Geometry: final body of the model. Coordinates: model frame, mm. Round coordinates to 2 decimals unless told otherwise and drop trailing zeros. Loops run counter-clockwise (first coordinate to the right, second up) from the corner with the lowest first, then second, coordinate; pieces in that order, holes last. Notation, with made-up numbers: M 65,35 L 92,35 A18 cw 92,51 Z; hole C -34,35.25 d7. An arc over 180 degrees is marked long. Return JSON: item names as keys, results as strings.
from build123d import *

# Parameters (mm, degrees)
F1_DEPTH  = 4
F3_DEPTH  = 2
F5_DEPTH  = 2
F6_W      = 5
F6_H      = 4
F6_W_2    = 4
F6_H_2    = 5
F7_DEPTH  = 2
F9_R      = 5
F10_DEPTH = 4.001


with BuildPart() as f1:
    # F0 (on Top) → F1 (new body)
    with BuildSketch(Plane.XY):
        with BuildLine():
            ThreePointArc((51.5, 24), (48.5710678119, 31.0710678119), (41.5, 34))
            Line((41.5, 34), (-41.5, 34))
            ThreePointArc((-41.5, 34), (-48.5710678119, 31.0710678119), (-51.5, 24))
            Line((-51.5, 24), (-51.5, -24))
            ThreePointArc((-51.5, -24), (-48.5710678119, -31.0710678119), (-41.5, -34))
            Line((-41.5, -34), (41.5, -34))
            ThreePointArc((41.5, -34), (48.5710678119, -31.0710678119), (51.5, -24))
            Line((51.5, -24), (51.5, 24))
        make_face()
        with BuildLine():
            ThreePointArc((41.5, 30), (45.7426406871, 28.2426406871), (47.5, 24))
            Line((47.5, 24), (47.5, -24))
            ThreePointArc((47.5, -24), (45.7426406871, -28.2426406871), (41.5, -30))
            Line((41.5, -30), (-41.5, -30))
            ThreePointArc((-41.5, -30), (-45.7426406871, -28.2426406871), (-47.5, -24))
            Line((-47.5, -24), (-47.5, 24))
            ThreePointArc((-47.5, 24), (-45.7426406871, 28.2426406871), (-41.5, 30))
            Line((-41.5, 30), (41.5, 30))
        make_face(mode=Mode.SUBTRACT)
    extrude(amount=F1_DEPTH)

    # F2 (on face) → F5 (join)
    with BuildSketch(Plane.XY.offset(4)):
        with BuildLine():
            ThreePointArc((51.5, 24), (48.5710678119, 31.0710678119), (41.5, 34))
            Line((41.5, 34), (-41.5, 34))
            ThreePointArc((-41.5, 34), (-48.5710678119, 31.0710678119), (-51.5, 24))
            Line((-51.5, 24), (-51.5, -24))
            ThreePointArc((-51.5, -24), (-48.5710678119, -31.0710678119), (-41.5, -34))
            Line((-41.5, -34), (41.5, -34))
            ThreePointArc((41.5, -34), (48.5710678119, -31.0710678119), (51.5, -24))
            Line((51.5, -24), (51.5, 24))
        make_face()
        with BuildLine():
            Line((-41.5, 30), (41.5, 30))
            ThreePointArc((41.5, 30), (45.7426406871, 28.2426406871), (47.5, 24))
            Line((47.5, 24), (47.5, -24))
            ThreePointArc((47.5, -24), (45.7426406871, -28.2426406871), (41.5, -30))
            Line((41.5, -30), (-41.5, -30))
            ThreePointArc((-41.5, -30), (-45.7426406871, -28.2426406871), (-47.5, -24))
            Line((-47.5, -24), (-47.5, 24))
            ThreePointArc((-47.5, 24), (-45.7426406871, 28.2426406871), (-41.5, 30))
        make_face(mode=Mode.SUBTRACT)
        with BuildLine():
            ThreePointArc((47.5, 24), (45.7426406871, 28.2426406871), (41.5, 30))
            Line((41.5, 30), (-41.5, 30))
            ThreePointArc((-41.5, 30), (-45.7426406871, 28.2426406871), (-47.5, 24))
            Line((-47.5, 24), (-47.5, -24))
            ThreePointArc((-47.5, -24), (-45.7426406871, -28.2426406871), (-41.5, -30))
            Line((-41.5, -30), (41.5, -30))
            ThreePointArc((41.5, -30), (45.7426406871, -28.2426406871), (47.5, -24))
            Line((47.5, -24), (47.5, 24))
        make_face()
    extrude(amount=-F5_DEPTH)

    # F6 (on face) → F7 (cut)
    with BuildSketch(Plane(origin=(0, 0, 0), x_dir=(1, 0, 0), z_dir=(0, 0, -1))):
        with Locations((-35.85, 32)):
            Rectangle(F6_W, F6_H)
        with Locations((35.85, 32)):
            Rectangle(F6_W, F6_H)
        with Locations((-35.85, -32)):
            Rectangle(F6_W, F6_H)
        with Locations((35.85, -32)):
            Rectangle(F6_W, F6_H)
        with Locations((-49.5, 20)):
            Rectangle(F6_W_2, F6_H_2)
        with Locations((-49.5, -20)):
            Rectangle(F6_W_2, F6_H_2)
        with Locations((49.5, -20)):
            Rectangle(F6_W_2, F6_H_2)
        with Locations((49.5, 20)):
            Rectangle(F6_W_2, F6_H_2)
    extrude(amount=-F7_DEPTH, mode=Mode.SUBTRACT)

    # F9 (on face) → F10 (cut, through all)
    with BuildSketch(Plane.XY.offset(4)):
        with Locations((-42.4, 24)):
            Circle(F9_R)
        with BuildLine():
            Line((-26.8, 30), (-36.8, 30))
            ThreePointArc((-36.8, 30), (-31.8, 25), (-26.8, 30))
        make_face()
        with Locations((-31.8, 18)):
            Circle(F9_R)
        with Locations((-42.4, 12)):
            Circle(F9_R)
        with Locations((-42.4, 0)):
            Circle(F9_R)
        with Locations((-31.8, 6)):
            Circle(F9_R)
        with Locations((-31.8, -6)):
            Circle(F9_R)
        with Locations((-42.4, -12)):
            Circle(F9_R)
        with Locations((-42.4, -24)):
            Circle(F9_R)
        with Locations((-31.8, -18)):
            Circle(F9_R)
        with BuildLine():
            ThreePointArc((-26.8, -30), (-31.8, -25), (-36.8, -30))
            Line((-36.8, -30), (-26.8, -30))
        make_face()
        with Locations((-21.2, -24)):
            Circle(F9_R)
        with Locations((-21.2, -12)):
            Circle(F9_R)
        with Locations((-21.2, 0)):
            Circle(F9_R)
        with Locations((-21.2, 12)):
            Circle(F9_R)
        with Locations((-21.2, 24)):
            Circle(F9_R)
        with BuildLine():
            ThreePointArc((-15.6, 30), (-10.6, 25), (-5.6, 30))
            Line((-5.6, 30), (-15.6, 30))
        make_face()
        with Locations((-10.6, 18)):
            Circle(F9_R)
        with Locations((-10.6, 6)):
            Circle(F9_R)
        with Locations((-10.6, -6)):
            Circle(F9_R)
        with Locations((-10.6, -18)):
            Circle(F9_R)
        with BuildLine():
            Line((-15.6, -30), (-5.6, -30))
            ThreePointArc((-5.6, -30), (-10.6, -25), (-15.6, -30))
        make_face()
        with Locations((0, -24)):
            Circle(F9_R)
        with Locations((0, -12)):
            Circle(F9_R)
        Circle(F9_R)
        with Locations((0, 12)):
            Circle(F9_R)
        with Locations((0, 24)):
            Circle(F9_R)
        with BuildLine():
            Line((15.6, 30), (5.6, 30))
            ThreePointArc((5.6, 30), (10.6, 25), (15.6, 30))
        make_face()
        with Locations((10.6, 18)):
            Circle(F9_R)
        with Locations((10.6, 6)):
            Circle(F9_R)
        with Locations((10.6, -6)):
            Circle(F9_R)
        with Locations((10.6, -18)):
            Circle(F9_R)
        with BuildLine():
            ThreePointArc((15.6, -30), (10.6, -25), (5.6, -30))
            Line((5.6, -30), (15.6, -30))
        make_face()
        with Locations((21.2, -24)):
            Circle(F9_R)
        with Locations((21.2, -12)):
            Circle(F9_R)
        with Locations((21.2, 0)):
            Circle(F9_R)
        with Locations((21.2, 12)):
            Circle(F9_R)
        with Locations((21.2, 24)):
            Circle(F9_R)
        with BuildLine():
            ThreePointArc((26.8, 30), (31.8, 25), (36.8, 30))
            Line((36.8, 30), (26.8, 30))
        make_face()
        with Locations((31.8, 18)):
            Circle(F9_R)
        with Locations((31.8, 6)):
            Circle(F9_R)
        with Locations((31.8, -6)):
            Circle(F9_R)
        with Locations((31.8, -18)):
            Circle(F9_R)
        with BuildLine():
            Line((26.8, -30), (36.8, -30))
            ThreePointArc((36.8, -30), (31.8, -25), (26.8, -30))
        make_face()
        with Locations((42.4, -24)):
            Circle(F9_R)
        with Locations((42.4, -12)):
            Circle(F9_R)
        with Locations((42.4, 0)):
            Circle(F9_R)
        with Locations((42.4, 12)):
            Circle(F9_R)
        with Locations((42.4, 24)):
            Circle(F9_R)
    extrude(amount=-F10_DEPTH, mode=Mode.SUBTRACT)


with BuildPart() as f3:
    # F2 (on face) → F3 (new body)
    with BuildSketch(Plane.XY.offset(4)):
        with BuildLine():
            ThreePointArc((51.5, 24), (48.5710678119, 31.0710678119), (41.5, 34))
            Line((41.5, 34), (-41.5, 34))
            ThreePointArc((-41.5, 34), (-48.5710678119, 31.0710678119), (-51.5, 24))
            Line((-51.5, 24), (-51.5, -24))
            ThreePointArc((-51.5, -24), (-48.5710678119, -31.0710678119), (-41.5, -34))
            Line((-41.5, -34), (41.5, -34))
            ThreePointArc((41.5, -34), (48.5710678119, -31.0710678119), (51.5, -24))
            Line((51.5, -24), (51.5, 24))
        make_face()
        with BuildLine():
            Line((-41.5, 30), (41.5, 30))
            ThreePointArc((41.5, 30), (45.7426406871, 28.2426406871), (47.5, 24))
            Line((47.5, 24), (47.5, -24))
            ThreePointArc((47.5, -24), (45.7426406871, -28.2426406871), (41.5, -30))
            Line((41.5, -30), (-41.5, -30))
            ThreePointArc((-41.5, -30), (-45.7426406871, -28.2426406871), (-47.5, -24))
            Line((-47.5, -24), (-47.5, 24))
            ThreePointArc((-47.5, 24), (-45.7426406871, 28.2426406871), (-41.5, 30))
        make_face(mode=Mode.SUBTRACT)
    extrude(amount=-F3_DEPTH)


solid = f1.part
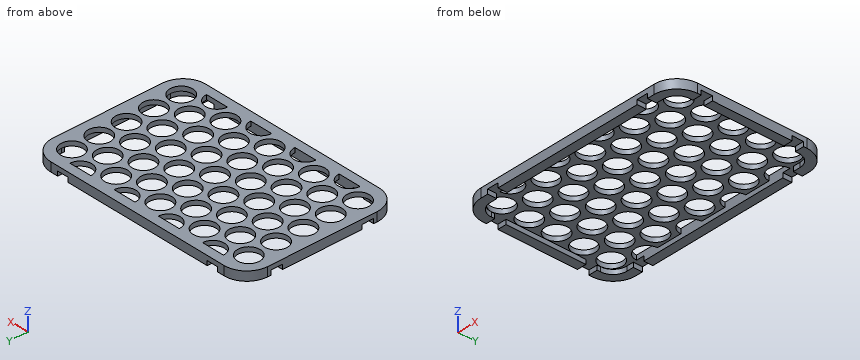
Q1. Pin query (flat end, axial travel): pin 1 (1.6 mm diameter, centred on x = -49, z = 0.5, fed in from +Y); pin 2 (4 mm diameter, centred on x = 13.5, y = -21.5, fed in from -Z); pin 3 (1 mm diameter, centred on x = -50.5, z = 0.5, fed in from -Y). Return the tip coordinate at first contact, or that it passes through.
Determined:
{"pin 1": "stops at y = 31.42", "pin 2": "stops at z = 2", "pin 3": "stops at y = -29.27"}
Q2. Section query B-B (x = -10.6). Output: boundary loops of the cut face in (y, z), plus the area to 3 significant figures.
Determined:
{"outline": "M -34,0 L -30,0 L -30,4 L -34,4 Z; M -25,2 L -23,2 L -23,4 L -25,4 Z; M -13,2 L -11,2 L -11,4 L -13,4 Z; M -1,2 L 1,2 L 1,4 L -1,4 Z; M 11,2 L 13,2 L 13,4 L 11,4 Z; M 23,2 L 25,2 L 25,4 L 23,4 Z; M 30,0 L 34,0 L 34,4 L 30,4 Z", "area": "52.0 mm^2"}
Q3. Section query C-C (x = -21.2). Output: boundary loops of the cut face in (y, z), plus the area to 3 significant figures.
Determined:
{"outline": "M -34,0 L -30,0 L -30,2 L -29,2 L -29,4 L -34,4 Z; M -19,2 L -17,2 L -17,4 L -19,4 Z; M -7,2 L -5,2 L -5,4 L -7,4 Z; M 5,2 L 7,2 L 7,4 L 5,4 Z; M 17,2 L 19,2 L 19,4 L 17,4 Z; M 29,2 L 30,2 L 30,0 L 34,0 L 34,4 L 29,4 Z", "area": "52.0 mm^2"}
Q4. Section query A-A (y = -6). Output: boundary loops of the cut face in (x, z), plus the area to 3 significant figures.
Determined:
{"outline": "M -51.5,0 L -47.5,0 L -47.5,2 L -36.8,2 L -36.8,4 L -51.5,4 Z; M -26.8,2 L -15.6,2 L -15.6,4 L -26.8,4 Z; M -5.6,2 L 5.6,2 L 5.6,4 L -5.6,4 Z; M 15.6,2 L 26.8,2 L 26.8,4 L 15.6,4 Z; M 36.8,2 L 47.5,2 L 47.5,0 L 51.5,0 L 51.5,4 L 36.8,4 Z", "area": "142 mm^2"}
Q5. Section query D-D (z = 2.8). State how many separate pieces and enclosed holes the cut face has, plus the area to 3 significant figures.
Determined:
{"separate pieces": "1", "enclosed holes": "49", "area": "3,380 mm^2"}
Q6. Material intervals for L1, parallel to X at y = 24.5, z = 2.5; L2, parallel to Y at x = -21.2, z = 3; L3, parallel to Y at x = -30, z = 1.3, sorted ascending.
Determined:
{"L1": "x = -51.49 to -47.37, -37.43 to -26.17, -16.23 to -4.97, 4.97 to 16.23, 26.17 to 37.43, 47.37 to 51.49", "L2": "y = -34 to -29, -19 to -17, -7 to -5, 5 to 7, 17 to 19, 29 to 34", "L3": "y = -34 to -30, 30 to 34"}
